Autodesk Fusion 360 part; units mm, degrees
sketch "Sketch1" plane through (0, 0, 0) normal (0, 0, 1) x (1, 0, 0)
  line L0 (0, 0) -> (32, 0)
  line L1 (32, 0) -> (32, -6)
  line L2 (32, -6) -> (0, -6)
  line L3 (0, -6) -> (0, 0)
  circle A0 centre (36.0053, -3) radius 4
  line L4 (32, 0) -> (33.3595, 0)
  line L5 (32, -6) -> (33.3595, -6)
  dimension "d1" = 32
  dimension "d2" = 6
  dimension "d3" = 8
extrude "Extrude1" add sketch "Sketch1" along normal blind 4 contours L0 L1 L2 L3 | L1 A0 L4 L5
extrude "Extrude2" add sketch "Sketch1" along normal blind 5.5 contours A0
hole "Hole1" at (36.0053, -3, 5.5) direction (0, 0, -1) diameter 6.2 depth 4 tip angle 180
sketch "Sketch2" plane through (0, 0, 5.5) normal (0, 0, 1) x (-1, 0, 0)
  circle A0 centre (-36.0053, 3) radius 3.1
  circle A1 centre (-36.0053, 3) radius 4
  arc A2 (-36.0053, 6.1) -> (-36.0053, -0.1) centre (-35.6842, 3) ccw
extrude "Extrude3" add sketch "Sketch2" against normal blind 0.5 contours A0 A2 picked at (-36.835, 3.299)
mirror "Mirror1" about plane through (0, -6, 0) normal (-1, 0, 0) of bodies 1 merged
Work out the finished part from the listing and answer in its coordinate system (mm). Give positions to 0.01 mm unless a question says otherwise; leave off trailing zeros. Loops run counter-clockwise (first coordinate to the right, second up) from the corner with the lowest first, then second, coordinate; pieces in that order, holes last. Notation, with made-up numbers: (-31.5, 24.5) - (-9.5, 24.5) arc R19 cw to (-9.5, 59.5) - close; hole circle Ø7 at (79.25, 0). An arc over 180 degrees is marked (long way). One line per question, with ' | ' between items.
(1) The part is cut by section A-A (z = 2.75). Write down the section's boundary in (x, y).
Recorded:
outline: (-33.36, -6) - (33.36, -6) arc R4 ccw (long way) to (33.36, 0) - (-33.36, 0) arc R4 ccw (long way) to start; hole circle Ø6.2 at (-36.01, -3); hole circle Ø6.2 at (36.01, -3)
(2) The part is cut by section B-B (x = -16). Write down the section's boundary in (y, z), then the cut area to 3 significant figures.
Recorded:
outline: (-6, 0) - (0, 0) - (0, 4) - (-6, 4) - close | area: 24.0 mm²
(3) Straight lines are drawn through the part: probe 1 along X at (y, z) = (-3, 2.4); probe 2 along X at (y, z) = (-3, 4.3); probe 3 along Z at (x, y) = (36.5, -1.5). For each, find the intervals that lie inside material, in ascending order.
Recorded:
probe 1: x = -40.01 to -39.11, -32.91 to 32.91, 39.11 to 40.01 | probe 2: x = -40.01 to -39.11, -32.91 to -32.01, 32.01 to 32.91, 39.11 to 40.01 | probe 3: z = 0 to 1.5, 5 to 5.5
(4) Each of these flat-tipped pins is pushed along its axis until it touches: pin 1 Ø3 at (x, z) = (17, 1) entering from -Y; pin 2 Ø0.7 at (x, z) = (32.5, 3) entering from +Y. Where does it stop, or does it pass through?
Recorded:
pin 1: stops at y = -6 | pin 2: stops at y = 0
